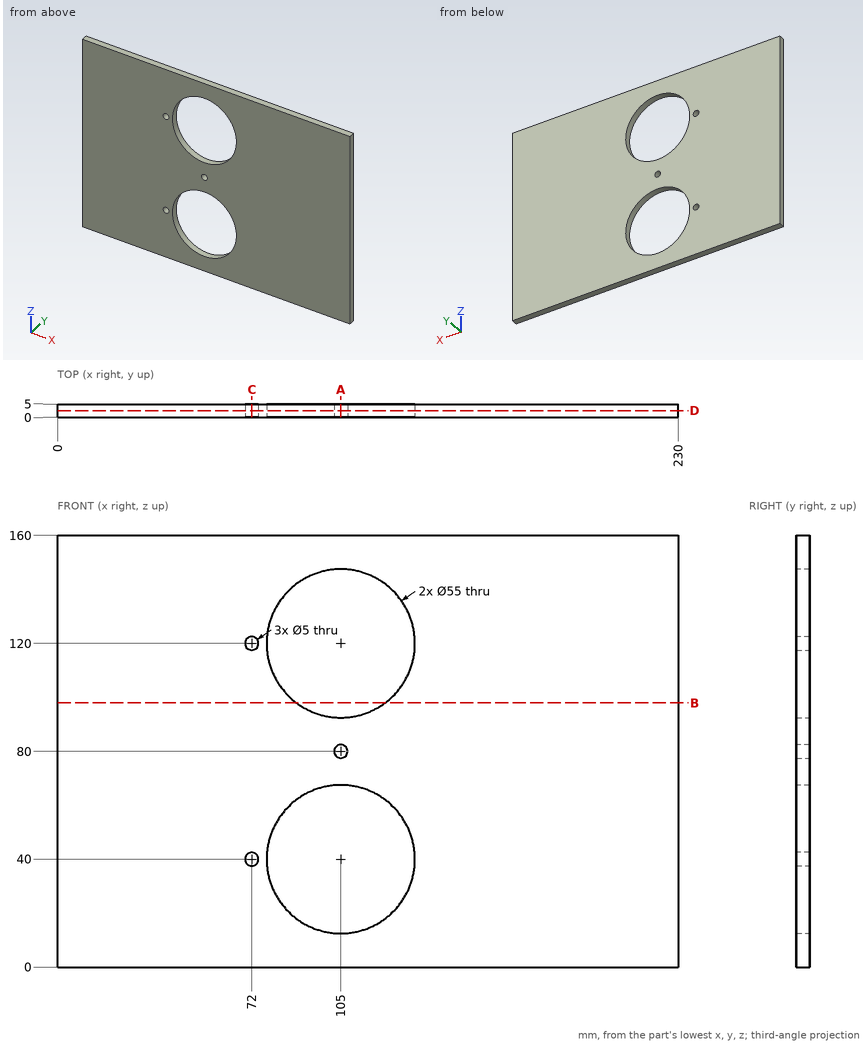
Geometry: see drawing. Coordinates: mm, zero at the bounding-box minimum. Give positions to 0.01 mm unless a question says otherwise; leave off trailing zeros. Order: outer loops, then holes, each group sorted by start corner. A loop starts at its lowest first (then second) coordinate and runs counter-clockwise, first axis right, second up. Notation, with made-up numbers: (0.25, 48.5) - (58.25, 48.5) arc R24 cw to (58.25, 62.5) - close; hole circle Ø6 at (20, 6). An arc over 180 degrees is marked (long way). Use CSV: the item, a comma, the result in double quotes.
1. Section query C-C (x = 72). Output: boundary loops of the cut face in (y, z).
Answers below:
outline,"(0, 0) - (5, 0) - (5, 37.5) - (0, 37.5) - close; (0, 42.5) - (5, 42.5) - (5, 117.5) - (0, 117.5) - close; (0, 122.5) - (5, 122.5) - (5, 160) - (0, 160) - close"
2. Section query B-B (z = 98). Output: boundary loops of the cut face in (x, y).
Answers below:
outline,"(0, 0) - (88.5, 0) - (88.5, 5) - (0, 5) - close; (121.5, 0) - (230, 0) - (230, 5) - (121.5, 5) - close"
3. Material intervals for line 1 along X through (y, z) = (3.95, 40); line 2 along X through (y, z) = (3, 80); line 3 along Z through (x, y) = (130, 0.3), sorted ascending. Write a range as from..to.
Answers below:
line 1,"0..69.5, 74.5..77.5, 132.5..230"
line 2,"0..102.5, 107.5..230"
line 3,"0..28.54, 51.46..108.54, 131.46..160"
4. Section query A-A (x = 105). Output: boundary loops of the cut face in (y, z).
Answers below:
outline,"(0, 0) - (5, 0) - (5, 12.5) - (0, 12.5) - close; (0, 67.5) - (5, 67.5) - (5, 77.5) - (0, 77.5) - close; (0, 82.5) - (5, 82.5) - (5, 92.5) - (0, 92.5) - close; (0, 147.5) - (5, 147.5) - (5, 160) - (0, 160) - close"
5. Section query D-D (y = 2.55). Output: boundary loops of the cut face in (x, z).
Answers below:
outline,"(0, 0) - (230, 0) - (230, 160) - (0, 160) - close; hole circle Ø5 at (72, 40); hole circle Ø5 at (72, 120); hole circle Ø55 at (105, 40); hole circle Ø55 at (105, 120); hole circle Ø5 at (105, 80)"
